```python
from build123d import *

# Parameters (mm, degrees)
F0_W     = 220.6
F0_H     = 305.7
F1_DEPTH = 9
F2_W     = 196.6
F2_H     = 262.7
F3_DEPTH = 1
F4_R     = 2.5
F4_R_2   = 5
F5_DEPTH = 1
F6_R     = 5
F7_R     = 1


with BuildPart() as f1:
    # F0 (on Front) → F1 (new body)
    with BuildSketch(Plane.XZ):
        with Locations((0, 152.85)):
            Rectangle(F0_W, F0_H)
    extrude(amount=F1_DEPTH)

    # F2 (on face) → F3 (cut)
    with BuildSketch(Plane.XZ.offset(9)):
        with Locations((0, 152.85)):
            Rectangle(F2_W, F2_H)
    extrude(amount=-F3_DEPTH, mode=Mode.SUBTRACT)

    # F4 (on face) → F5 (cut)
    with BuildSketch(Plane.XZ.offset(9)):
        with Locations((0, 295.7)):
            Circle(F4_R)
        with Locations((0, 11)):
            Circle(F4_R_2)
    extrude(amount=-F5_DEPTH, mode=Mode.SUBTRACT)

    # F6
    f6_edges = [f1.edges().sort_by_distance(p)[0] for p in [
        (-110.3, -4.5, 0),
        (110.3, -4.5, 0),
        (110.3, -4.5, 305.7),
        (-110.3, -4.5, 305.7),
    ]]
    fillet(f6_edges, radius=F6_R)

    # F7
    f7_edges = [f1.edges().sort_by_distance(p)[0] for p in [
        (-110.3, -9, 152.85),
        (-110.3, 0, 152.85),
    ]]
    fillet(f7_edges, radius=F7_R)


solid = f1.part
```
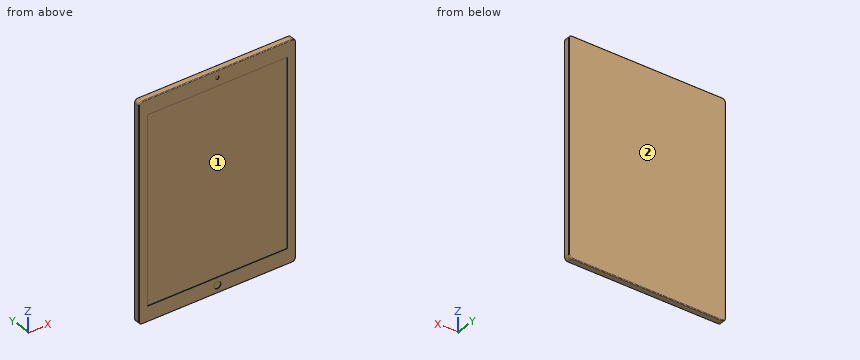
Read the model definition and answer for the solid it produces. Units are mm, in the model's axes. Face numbers are marked on the shaded views. Give positions to 0.01 mm unless a question says otherwise; leave off trailing zeros. Write each loop counter-clockwise with the first axis right and the second up, starting at its lowest first coordinate (ties: lowest second). Pieces come first, ordered by that corner, then holes. Notation, with made-up numbers: (65, 25) -> (109, 25) arc R20 cw to (109, 63) -> close; hole circle Ø11 at (27.5, 64). An arc over 180 degrees is marked (long way). Answer as a JSON object with one key per item and string values.
1) Section B-B on z = 259 is taken. Write down the section's boundary in (x, y), then the cut area to 3 significant figures.
Findings below:
{"outline": "(-110.3, -8) arc R1 ccw to (-109.3, -9) -> (-98.3, -9) -> (-98.3, -8) -> (98.3, -8) -> (98.3, -9) -> (109.3, -9) arc R1 ccw to (110.3, -8) -> (110.3, -1) arc R1 ccw to (109.3, 0) -> (-109.3, 0) arc R1 ccw to (-110.3, -1) -> close", "area": "1,790 mm^2"}
2) Flat-ended cylindrical pins translate along their axes: pin 1 Ø1.5 at (x, z) = (49, 154.5) entering from -Y; pin 2 Ø0.8 at (x, y) = (27, -8.5) entering from +Z (3 decimals); pin 3 Ø0.5 at (y, z) = (-8.5, 154.5) entering from +X. Find the tip coordinate at first contact, or state that the pin passes through.
Findings below:
{"pin 1": "stops at y = -8", "pin 2": "stops at z = 305.695", "pin 3": "stops at x = 110.27"}
3) Section A-A on x = -32 is taken. Write down the section's boundary in (y, z), then the cut area to 3 significant figures.
Findings below:
{"outline": "(-9, 1) arc R1 ccw to (-8, 0) -> (-1, 0) arc R1 ccw to (0, 1) -> (0, 304.7) arc R1 ccw to (-1, 305.7) -> (-8, 305.7) arc R1 ccw to (-9, 304.7) -> (-9, 284.2) -> (-8, 284.2) -> (-8, 21.5) -> (-9, 21.5) -> close", "area": "2,490 mm^2"}
4) Straight lines are drawn through the part: probe 1 along Z at (x, y) = (0, -8.2); probe 2 along X at (y, z) = (-8.25, 103); probe 3 along Z at (x, y) = (0, -8.8). For each, find the intervals that lie inside material, in ascending order. Write a range as from..to.
Findings below:
{"probe 1": "z = 0.02..6, 16..21.5, 284.2..293.2, 298.2..305.68", "probe 2": "x = -110.27..-98.3, 98.3..110.27", "probe 3": "z = 0.4..6, 16..21.5, 284.2..293.2, 298.2..305.3"}
5) For a pull along X with two mould halves and no side action, classify the marked faces 1 and 2 as pulls with the +X half, pulls with the -X half, needs draft (parallel to the pull), parting line crosses it, or undercut.
Findings below:
{"face 1": "undercut", "face 2": "needs draft"}
